from build123d import *

# Parameters (mm, degrees)
PLATE_DEPTH           = 3
SKETCH2_R             = 6
MOUNT_POSTS_DEPTH     = 22
SKETCH3_R             = 4.25
MOUNT_CBORE_DEPTH     = 19.5
F_8_CLEARANCE_HOLE1_D = 4.4958
FILLET1_R             = 1.5
SKETCH7_R             = 1.9
TERMINAL_STRIP_DEPTH  = 166.90660023
SKETCH9_W             = 60
SKETCH9_H             = 12
WIRING_RELIEF_DEPTH   = 166.90660023
CHAMFER1_SIZE         = 3
CHAMFER2_SIZE         = 1
FILLET2_R             = 5
FILLET3_R             = 1.5


with BuildPart() as part:
    # Sketch1 → plate (new body)
    with BuildSketch(Plane(origin=(0, 0, 0), x_dir=(1, 0, 0), z_dir=(0, 1, 0))):
        Polygon((0, 0), (83, 0), (83, 65), (121, 65), (121, 110), (0, 110), align=None)
    extrude(amount=PLATE_DEPTH)

    # Sketch2 → mount posts (add)
    with BuildSketch(Plane(origin=(0, 3, 0), x_dir=(1, 0, 0), z_dir=(0, 1, 0))):
        with Locations(Location((75, 85.75, 0), (0, 0, 270))):
            Circle(SKETCH2_R)
        with Locations(Location((75, 24.25, 0), (0, 0, 270))):
            Circle(SKETCH2_R)
    extrude(amount=-MOUNT_POSTS_DEPTH)

    # Sketch3 → mount cbore (cut)
    with BuildSketch(Plane(origin=(0, 3, 0), x_dir=(1, 0, 0), z_dir=(0, 1, 0))):
        with Locations(Location((75, 85.75, 0), (0, 0, 270))):
            Circle(SKETCH3_R)
        with Locations(Location((75, 24.25, 0), (0, 0, 270))):
            Circle(SKETCH3_R)
    extrude(amount=-MOUNT_CBORE_DEPTH, mode=Mode.SUBTRACT)

    # #8 Clearance Hole1 (through all)
    with Locations(Plane(origin=(0, -16.5, 0), x_dir=(1, 0, 0), z_dir=(0, 1, 0))):
        with Locations((75, 85.75), (75, 24.25)):
            Hole(F_8_CLEARANCE_HOLE1_D / 2)

    # Sketch8 → foot (revolve)
    with BuildSketch(Plane(origin=(0, 0, -55), x_dir=(1, 0, 0), z_dir=(0, 0, -1)), mode=Mode.PRIVATE) as foot_sk:
        Polygon((47.25, 0), (48.85, 0), (47.1, 25), (45.5, 25), align=None)
    revolve(foot_sk.sketch.rotate(Axis((42, 0, -55), (0, -1, 0)), 90), axis=Axis((42, 0, -55), (0, -1, 0)))

    # Fillet1
    fillet1_edges = [part.edges().sort_by_distance(p)[0] for p in [
        (42, 0, -60.25),
        (42, 0, -61.85),
    ]]
    fillet(fillet1_edges, radius=FILLET1_R)

    # Sketch7 → terminal strip (cut, through all)
    with BuildSketch(Plane(origin=(0, 3, 0), x_dir=(1, 0, 0), z_dir=(0, 1, 0))):
        with Locations(Location((115.34, 97, 0), (0, 0, 270))):
            Circle(SKETCH7_R)
        with Locations(Location((86.66, 97, 0), (0, 0, 270))):
            Circle(SKETCH7_R)
        with BuildLine():
            Line((96.2375, 101.5), (105.7625, 101.5))
            ThreePointArc((105.7625, 101.5), (110.2625, 97), (105.7625, 92.5))
            Line((105.7625, 92.5), (96.2375, 92.5))
            ThreePointArc((96.2375, 92.5), (91.7375, 97), (96.2375, 101.5))
        make_face()
    extrude(amount=-TERMINAL_STRIP_DEPTH, mode=Mode.SUBTRACT)

    # Sketch9 → wiring relief (cut, through all)
    with BuildSketch(Plane(origin=(0, 3, 0), x_dir=(1, 0, 0), z_dir=(0, 1, 0))):
        with Locations((30, 104)):
            Rectangle(SKETCH9_W, SKETCH9_H)
    extrude(amount=-WIRING_RELIEF_DEPTH, mode=Mode.SUBTRACT)

    # Chamfer1
    # the kernel refuses this chamfer: 3 mm, written as the material it adds along each edge
    with BuildSketch(Plane(origin=(75, -16.5, -85.75), x_dir=(0, 0, 1), z_dir=(-1, 0, 0))) as chamfer1_piece_1_section:
        Polygon((4.25, CHAMFER1_SIZE), (4.25 - CHAMFER1_SIZE, 0), (4.25, 0), align=None)
    chamfer1_piece_1 = revolve(axis=Axis((75, -16.5, -85.75), (0, 1, 0)), mode=Mode.PRIVATE)
    chamfer1_piece_1 = chamfer1_piece_1 - Plane(origin=(75, -14.490807126, -85.75), x_dir=(-1, 0, 0), z_dir=(0, -1, 0)) * Cylinder(2.2479, 17, mode=Mode.PRIVATE)
    add(chamfer1_piece_1)
    with BuildSketch(Plane(origin=(75, -16.5, -24.25), x_dir=(0, 0, 1), z_dir=(-1, 0, 0))) as chamfer1_piece_2_section:
        Polygon((4.25, CHAMFER1_SIZE), (4.25 - CHAMFER1_SIZE, 0), (4.25, 0), align=None)
    chamfer1_piece_2 = revolve(axis=Axis((75, -16.5, -24.25), (0, 1, 0)), mode=Mode.PRIVATE)
    chamfer1_piece_2 = chamfer1_piece_2 - Plane(origin=(75, -14.490807126, -24.25), x_dir=(-1, 0, 0), z_dir=(0, -1, 0)) * Cylinder(2.2479, 18, mode=Mode.PRIVATE)
    add(chamfer1_piece_2)

    # Chamfer2
    chamfer2_edges = [part.edges().sort_by_distance(p)[0] for p in [
        (75, -19, -91.75),
        (75, -19, -30.25),
    ]]
    chamfer(chamfer2_edges, length=CHAMFER2_SIZE)

    # Fillet2
    fillet2_edges = [part.edges().sort_by_distance(p)[0] for p in [
        (121, 1.5, -110),
        (121, 1.5, -65),
        (83, 1.5, -65),
        (83, 1.5, 0),
        (0, 1.5, 0),
        (0, 1.5, -98),
        (60, 1.5, -110),
        (60, 1.5, -98),
    ]]
    fillet(fillet2_edges, radius=FILLET2_R)

    # Fillet3
    fillet3_edges = [part.edges().sort_by_distance(p)[0] for p in [
        (75, 0, -91.75),
        (75, 0, -30.25),
    ]]
    fillet(fillet3_edges, radius=FILLET3_R)


solid = part.part
Design review of the part built by this model. Coordinates are the model's own, in mm. A direction names the side the tool comes from. Round coordinates to 2 decimals unless told otherwise and drop trailing zeros. Write each loop counter-clockwise with the first axis right and the second up, starting at its lowest first coordinate (ties: lowest second). Pieces come first, ordered by that corner, then holes. Notation, with made-up numbers: (45, 77) - (76, 77) arc R19 cw to (76, 87) - close; hole circle Ø4 at (-37, -30.5). An arc over 180 degrees is marked (long way). Use a Markdown table: item, result. Add a question column.
1. We need section A-A (z = -85.75). State the section outline as (x, y) points.
2. For faces 5 (the face through (110.26, 1.52, -97.1)), 6 (the face through (102, 1, -65)), 7 (the face through (43.66, -13.14, -51)), list the 3-axis set-ups (+Z, -Z, +X, -X, +Y, -Y) from which the entire face can be reached by the end or side of a thin tool; tool diameter is ignored.
3. We need section B-B (y = -6). State the section outline as (x, z) points.
4. Clearance check with flat-ended pins moving along their axes: pin 1 (6 mm diameter, centred on x = 75, z = -85.75, fed in from -Y); pin 2 (5 mm diameter, centred on y = -7.5, z = -56, fed in from -X); pin 3 (0.9 mm diameter, centred on x = 102.5, y = 1.5, fed in from +Z). State where each tip first meets the part, or that it passes through.
5. We need section D-D (z = -24.25). State the section outline as (x, y) points, then the cut area to 3 significant figures.
6. Mouldability with a two-part tool opening along X and no side actions: class faces 1 (the face through (91.74, 1.52, -96.9)), 2 (the face through (101, 2, -101.5)), 3 (the face through (1, 1, -96)), 4 (the face through (60, 0, -56)) as +X half, -X half, draft (parallel to the pull), parting line (faces both ways), or undercut.
7. Wall thickness on probe 1 along X at (y, z) = (2.15, -97); probe 2 along Z at (x, y) = (73.5, -1); probe 3 along X at (y, z) = (-17.3, -24.25): over which ranges is each line inside the solid? List them lowest first.
8. We need section C-C (x = 75). Count the separate pieces of the cut face and the enclosed holes in it, then the cut area to 3 significant figures.
Output:
| question | item | result |
|---|---|---|
| 1 | outline | (0, 0) - (67.5, 0) arc R1.5 cw to (69, -1.5) - (69, -18) - (70, -19) - (72.75, -19) - (72.75, -15.5) - (70.75, -13.5) - (70.75, 3) - (0, 3) - close; (77.25, -19) - (80, -19) - (81, -18) - (81, -1.5) arc R1.5 cw to (82.5, 0) - (121, 0) - (121, 3) - (79.25, 3) - (79.25, -13.5) - (77.25, -15.5) - close |
| 2 | face 5 | +Y, -Y |
| 2 | face 6 | +Z, +X, +Y, -Y |
| 2 | face 7 | none |
| 3 | outline | circle Ø12.86 at (42, -55); circle Ø12 at (75, -85.75); circle Ø12 at (75, -24.25); hole circle Ø9.66 at (42, -55); hole circle Ø8.5 at (75, -85.75); hole circle Ø8.5 at (75, -24.25) |
| 4 | pin 1 | stops at y = -19 |
| 4 | pin 2 | stops at x = 35.51 |
| 4 | pin 3 | stops at z = -65 |
| 5 | outline | (0, 0) - (67.5, 0) arc R1.5 cw to (69, -1.5) - (69, -18) - (70, -19) - (72.75, -19) - (72.75, -15.5) - (70.75, -13.5) - (70.75, 3) - (0, 3) - close; (77.25, -19) - (80, -19) - (81, -18) - (81, -1.5) arc R1.5 cw to (82.5, 0) - (83, 0) - (83, 3) - (79.25, 3) - (79.25, -13.5) - (77.25, -15.5) - close |
| 5 | area | 308 mm2 |
| 6 | face 1 | undercut |
| 6 | face 2 | undercut |
| 6 | face 3 | -X half |
| 6 | face 4 | draft |
| 7 | probe 1 | x = 2 to 84.76, 88.56 to 91.74, 110.26 to 113.44, 117.24 to 121 |
| 7 | probe 2 | z = -91.65 to -89.73, -81.77 to -79.85, -30.15 to -28.23, -20.27 to -18.35 |
| 7 | probe 3 | x = 69 to 72.75, 77.25 to 81 |
| 8 | separate pieces | 3 |
| 8 | enclosed holes | 0 |
| 8 | area | 448 mm2 |
